Could you check a few things on this model? Use its own coordinates, in mm. Coordinates: 2 decimals unless noted, no trailing zeros. Loops run counter-clockwise (first coordinate to the right, second up) from the corner with the lowest first, then second, coordinate; pieces in that order, holes last. Notation, with made-up numbers: M -19,18.5 L 16,18.5 A28 cw 16,54.5 Z; hole C -29.75,-28 d6. An arc over 180 degrees is marked long. Return JSON: item names as keys, results as strings. Group by question number.
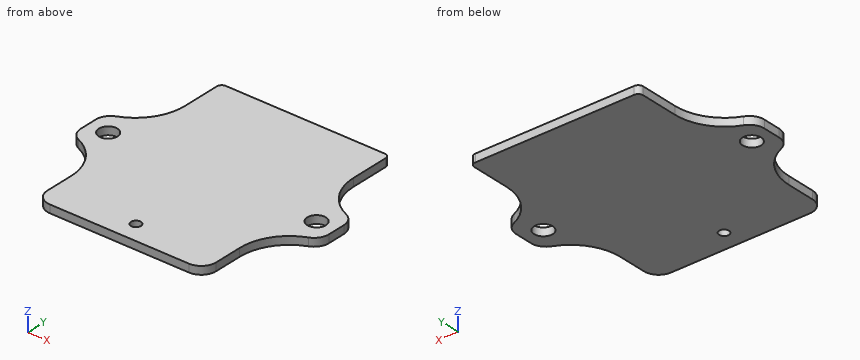
from build123d import *

# Parameters (mm, degrees)
SKETCH1_R           = 1
SKETCH1_R_2         = 1.875
BOSS_EXTRUDE1_DEPTH = 1.6


with BuildPart() as part:
    # Sketch1 → Boss-Extrude1 (new body)
    with BuildSketch(Plane.XY):
        with BuildLine():
            Line((30.883756862, 108.134882568), (30.883756862, 115.836923597))
            ThreePointArc((30.883756862, 115.836923597), (30.590863643, 116.544030379), (29.883756862, 116.836923597))
            Line((29.883756862, 116.836923597), (-2.116243138, 116.836923597))
            ThreePointArc((-2.116243138, 116.836923597), (-2.82334992, 116.544030379), (-3.116243138, 115.836923597))
            Line((-3.116243138, 115.836923597), (-3.116243138, 108.134882568))
            ThreePointArc((-3.116243138, 108.134882568), (-4.795740195, 102.587880606), (-9.270089292, 98.904113338))
            ThreePointArc((-9.270089292, 98.904113338), (-10.612394021, 97.798983157), (-11.116243138, 96.134882568))
            Line((-11.116243138, 96.134882568), (-11.116243138, 92.538964626))
            ThreePointArc((-11.116243138, 92.538964626), (-10.612394021, 90.874864038), (-9.270089292, 89.769733857))
            ThreePointArc((-9.270089292, 89.769733857), (-4.795740195, 86.085966588), (-3.116243138, 80.538964626))
            Line((-3.116243138, 80.538964626), (-3.116243138, 74.836923597))
            ThreePointArc((-3.116243138, 74.836923597), (-2.237563482, 72.715603254), (-0.116243138, 71.836923597))
            Line((-0.116243138, 71.836923597), (27.883756862, 71.836923597))
            ThreePointArc((27.883756862, 71.836923597), (30.005077205, 72.715603254), (30.883756862, 74.836923597))
            Line((30.883756862, 74.836923597), (30.883756862, 80.538964626))
            ThreePointArc((30.883756862, 80.538964626), (32.563253918, 86.085966588), (37.037603016, 89.769733857))
            ThreePointArc((37.037603016, 89.769733857), (38.379907745, 90.874864038), (38.883756862, 92.538964626))
            Line((38.883756862, 92.538964626), (38.883756862, 96.134882568))
            ThreePointArc((38.883756862, 96.134882568), (38.379907745, 97.798983157), (37.037603016, 98.904113338))
            ThreePointArc((37.037603016, 98.904113338), (32.563253918, 102.587880606), (30.883756862, 108.134882568))
        make_face()
        with Locations((13.883756862, 75.836923597)):
            Circle(SKETCH1_R, mode=Mode.SUBTRACT)
        with Locations((-7.116243138, 94.336923597)):
            Circle(SKETCH1_R_2, mode=Mode.SUBTRACT)
        with Locations((34.883756862, 94.336923597)):
            Circle(SKETCH1_R_2, mode=Mode.SUBTRACT)
    extrude(amount=BOSS_EXTRUDE1_DEPTH)


solid = part.part
(1) Imagine slicing it at A-A, the plane x = 14. Write out the boundary of the cut face in (y, z).
(2) Imagine slicing it at C-C, the plane y = 109.5. Write out the boundary of the cut face in (x, z), then the cut area to 3 significant figures.
(3) Will this pin go through, and if not, where does the flat tip stop? P1, Ø0.5, axis at y = 110.5, z = 0.5, coming from the -X side.
(4) If I drill on L1, parallel to X at y = 96, z = 0.8; L2, parallel to Y at x = 13, z = 1; L3, parallel to X at y = 75, z = 1, over which ranges is the centre line in solid material (lowest first)? Write a range as [from, to].
(5) Imagine slicing it at B-B, the plane z = 1.15. Write out the boundary of the cut face in (x, y) (3 decimals), then the cut area to 3 significant figures.
(6) Imagine slicing it at D-D, the plane x = 32. Write out the boundary of the cut face in (y, z).
Checks:
{
 "1": {"outline": "M 71.84,0 L 74.84,0 L 74.84,1.6 L 71.84,1.6 Z; M 76.83,0 L 116.84,0 L 116.84,1.6 L 76.83,1.6 Z"},
 "2": {"outline": "M -3.12,0 L 30.88,0 L 30.88,1.6 L -3.12,1.6 Z", "area": "54.4 mm²"},
 "3": {"P1": "x = -3.12"},
 "4": {"L1": "[-11.12, -7.98], [-6.25, 34.02], [35.75, 38.88]", "L2": "[71.84, 75.37], [76.3, 116.84]", "L3": "[-3.12, 13.34], [14.43, 30.88]"},
 "5": {"outline": "M -11.116,92.539 A3 ccw -9.27,89.77 A10 cw -3.116,80.539 L -3.116,74.837 A3 ccw -0.116,71.837 L 27.884,71.837 A3 ccw 30.884,74.837 L 30.884,80.539 A10 cw 37.038,89.77 A3 ccw 38.884,92.539 L 38.884,96.135 A3 ccw 37.038,98.904 A10 cw 30.884,108.135 L 30.884,115.837 A1 ccw 29.884,116.837 L -2.116,116.837 A1 ccw -3.116,115.837 L -3.116,108.135 A10 cw -9.27,98.904 A3 ccw -11.116,96.135 Z; hole C -7.116,94.337 d3.75; hole C 13.884,75.837 d2; hole C 34.884,94.337 d3.75", "area": "1,700 mm²"},
 "6": {"outline": "M 85.13,0 L 103.54,0 L 103.54,1.6 L 85.13,1.6 Z"}
}
